```python
from build123d import *

# Parameters (mm, degrees)
SKETCH1_W           = 30
SKETCH1_H           = 42
BOSS_EXTRUDE1_DEPTH = 7
SKETCH2_W           = 5.4
SKETCH2_H           = 40.4
CUT_EXTRUDE1_DEPTH  = 21
SKETCH3_W           = 5.4
SKETCH3_H           = 32
CUT_EXTRUDE2_DEPTH  = 21


with BuildPart() as part:
    # Sketch1 → Boss-Extrude1 (new body)
    with BuildSketch(Plane.XY):
        with Locations((15, 21)):
            Rectangle(SKETCH1_W, SKETCH1_H)
    extrude(amount=BOSS_EXTRUDE1_DEPTH)

    # Sketch2 → Cut-Extrude1 (cut)
    with BuildSketch(Plane.ZY):
        with Locations((3.5, 21)):
            Rectangle(SKETCH2_W, SKETCH2_H)
    extrude(amount=-CUT_EXTRUDE1_DEPTH, mode=Mode.SUBTRACT)

    # Sketch3 → Cut-Extrude2 (cut)
    with BuildSketch(Plane(origin=(30, 0, 0), x_dir=(0, 0, -1), z_dir=(1, 0, 0))):
        with Locations((-3.5, 21)):
            Rectangle(SKETCH3_W, SKETCH3_H)
    extrude(amount=-CUT_EXTRUDE2_DEPTH, mode=Mode.SUBTRACT)


solid = part.part
```
Verification items for the finished model (mm, model axes). A direction names the side the tool comes from. Coordinates: 2 decimals unless noted, no trailing zeros. Loops run counter-clockwise (first coordinate to the right, second up) from the corner with the lowest first, then second, coordinate; pieces in that order, holes last. Notation, with made-up numbers: (-25, 18.25) - (3, 18.25) arc R29 ccw to (3, 45.25) - close; hole circle Ø9 at (-20, -30). An arc over 180 degrees is marked (long way). Answer as a JSON object with one key per item and string values.
(1) Cross-section at D-D, the plane x = 2.5. Record the boundary of the cut face in (y, z), then the cut area to 3 significant figures.
Response:
{"outline": "(0, 0) - (42, 0) - (42, 7) - (0, 7) - close; hole (0.8, 0.8) - (41.2, 0.8) - (41.2, 6.2) - (0.8, 6.2) - close", "area": "75.8 mm²"}
(2) Mould release check, pull along Z, two halves, no side actions. Record for faces 4 (the flat face through (21, 39, 3)), 5 (the flat face through (15, 21, 7)), 6 (the flat face through (15, 42, 3)): pulls with the +Z half, pulls with the -Z half, needs draft (parallel to the pull), parting line crosses it, or undercut.
Response:
{"face 4": "undercut", "face 5": "pulls with the +Z half", "face 6": "needs draft"}
(3) Scan lines: line 1 along Z through (x, y) = (22.75, 6.5); line 2 along Y through (x, z) = (9.75, 3); line 3 along Y through (x, z) = (26.5, 3.75). Record each from-to range of solid material in increasing order.
Response:
{"line 1": "z = 0 to 0.8, 6.2 to 7", "line 2": "y = 0 to 0.8, 41.2 to 42", "line 3": "y = 0 to 5, 37 to 42"}
(4) Cross-section at C-C, the plane y = 28.5. Record the boundary of the cut face in (x, z), then the cut area to 3 significant figures.
Response:
{"outline": "(0, 0) - (30, 0) - (30, 0.8) - (0, 0.8) - close; (0, 6.2) - (30, 6.2) - (30, 7) - (0, 7) - close", "area": "48.0 mm²"}
(5) Go/stop test with a flat-tipped pin: pin 1 Ø3.5 at (y, z) = (38.5, 3) entering from -X. Record where the tip stops, or that it passes through.
Response:
{"pin 1": "stops at x = 21"}
(6) Cross-section at B-B, the plane x = 24. Record the boundary of the cut face in (y, z), then the cut area to 3 significant figures.
Response:
{"outline": "(0, 0) - (42, 0) - (42, 7) - (0, 7) - close; hole (5, 0.8) - (37, 0.8) - (37, 6.2) - (5, 6.2) - close", "area": "121 mm²"}
(7) Cross-section at A-A, the plane z = 2.25. Record the boundary of the cut face in (x, y), then the cut area to 3 significant figures.
Response:
{"outline": "(0, 0) - (30, 0) - (30, 5) - (21, 5) - (21, 0.8) - (0, 0.8) - close; (0, 41.2) - (21, 41.2) - (21, 37) - (30, 37) - (30, 42) - (0, 42) - close", "area": "124 mm²"}
(8) Access from +Z, -Z, +X, -X, +Y, -Y to the whole of each face (thin tool, end or side, straight path). Record for faces 1 (the flat face through (21, 3, 3)), 2 (the flat face through (26, 37, 4)), 3 (the flat face through (0, 19.3, 0.6)).
Response:
{"face 1": "-X", "face 2": "+X, -X", "face 3": "+Z, -Z, -X, +Y, -Y"}
